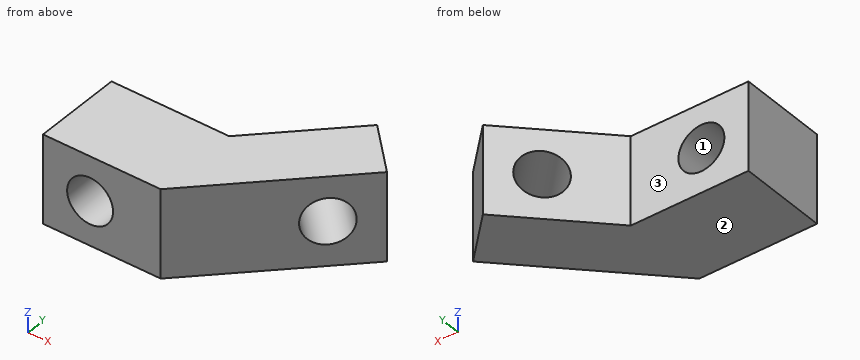
Autodesk Inventor part; units mm, degrees
ref_plane "YZ Plane" through (0, 0, 0) normal (1, 0, 0) x (0, 1, 0)
ref_plane "XZ Plane" through (0, 0, 0) normal (0, 1, 0) x (-1, 0, 0)
ref_plane "XY Plane" through (0, 0, 0) normal (0, 0, 1) x (1, 0, 0)
sketch "Sketch1" plane through (0, 0, 0) normal (0, 0, 1) x (1, 0, 0)
  line L0 (0, 0) -> (20, 0)
  line L1 (20, 0) -> (20, 15)
  line L2 (20, 15) -> (0, 15)
  line L3 (0, 15) -> (0, 0)
  dimension "d0" = 20
  dimension "d1" = 15
extrude "Extrusion1" add sketch "Sketch1" along normal blind 15
sketch "Sketch2" plane through (0, 15, 0) normal (0, 1, 0) x (1, 0, 0)
  line L0 (0, 0) -> (0, -15)
  circle A0 centre (8, -7.5) radius 3.9
  dimension "d4" = 7.8
  dimension "d6" = 8
extrude "Extrusion2" cut sketch "Sketch2" against normal blind 15
sketch "Sketch3" plane through (0, 0, 15) normal (0, 0, 1) x (1, 0, 0)
  line L0 (0, 0) -> (20, 0)
  line L1 (20, 0) -> (20, 15)
  line L2 (20, 0) -> (34.1421, 14.1421)
  line L3 (20, 15) -> (34.1421, 29.1421)
  line L4 (34.1421, 14.1421) -> (41.6421, 21.6421)
  line L5 (41.6421, 21.6421) -> (34.1421, 29.1421)
  dimension "d9" = 45
  dimension "d10" = 20
  dimension "d11" = 20
extrude "Extrusion3" add sketch "Sketch3" against normal blind 15
sketch "Sketch4" plane through (34.1421, 29.1421, 15) normal (-0.7071, 0.7071, 0) x (0.7071, 0.7071, 0)
  line L0 (0, 0) -> (0, 15)
  circle A0 centre (-8, 7.5) radius 3.9
  point P0 (-44.7487, 15)
  dimension "d14" = 7.8
  dimension "d16" = 8
extrude "Extrusion4" cut sketch "Sketch4" against normal blind 15
properties part number "connect stepper"
Input: part model. Units: mm. Frame: model coordinates. Face numbers are marked on the shaded views. Give positions to 0.01 mm unless a question says otherwise; leave off trailing zeros. Order: outer loops, then holes, each group sorted by start corner. A loop starts at its lowest first (then second) coordinate and runs counter-clockwise, first axis right, second up.
Q1. Section C-C on z = 9. Output: boundary loops of the cut face in (x, y).
Checked values:
outline: (0, 0) - (4.4, 0) - (4.4, 15) - (0, 15) - close; (11.6, 0) - (20, 0) - (33.44, 13.44) - (25.94, 20.94) - (20, 15) - (11.6, 15) - close; (31.03, 26.03) - (38.53, 18.53) - (41.64, 21.64) - (34.14, 29.14) - close
Q2. Section B-B on y = 2.5. Output: boundary loops of the cut face in (x, z).
Checked values:
outline: (0, 0) - (22.5, 0) - (22.5, 15) - (0, 15) - close; hole circle Ø7.8 at (8, 7.5)
Q3. Section A-A on x = 8. Output: boundary loops of the cut face in (y, z), and give its area (3 significant figures).
Checked values:
outline: (0, 0) - (15, 0) - (15, 3.6) - (0, 3.6) - close; (0, 11.4) - (15, 11.4) - (15, 15) - (0, 15) - close
area: 108 mm2
Q4. Draft query along Z for the marked faces 1, 2 and 3. Return one class per face: +Z half, -Z half, draft (parallel to the pull), parting line (faces both ways), or undercut.
Checked values:
face 1: undercut
face 2: -Z half
face 3: draft
Q5. Ray query, probe 1 along Z at (x, y) = (34, 18.25); probe 2 along Y at (x, z) = (3.5, 12.5); probe 3 along X at (y, z) = (8.5, 7.5). Return the intervals inside material, ascending.
Checked values:
probe 1: z = 0 to 3.61, 11.39 to 15
probe 2: y = 0 to 15
probe 3: x = 0 to 4.1, 11.9 to 28.5
Q6. Section D-D on z = 13. Output: boundary loops of the cut face in (x, y), and give its area (3 significant figures).
Checked values:
outline: (0, 0) - (20, 0) - (41.64, 21.64) - (34.14, 29.14) - (20, 15) - (0, 15) - close
area: 568 mm2
Q7. Contact query for flat-ended pins moving along their axis: pin 1 Ø8 at (x, z) = (31.5, 10) entering from -Y; pin 2 Ø8 at (y, z) = (3.5, 3.5) entering from +X; pin 3 Ø1 at (y, z) = (15.5, 12) entering from +X. Output: stop coordinate, or through.
Checked values:
pin 1: stops at y = 7.5
pin 2: stops at x = 27.5
pin 3: stops at x = 36
